The model under review builds one solid part; all positions refer to its coordinate system, in mm. Round coordinates to 2 decimals unless told otherwise and drop trailing zeros. Write each loop counter-clockwise with the first axis right and the second up, starting at its lowest first coordinate (ties: lowest second). Pieces come first, ordered by that corner, then holes.
Item 1: Add section A-A (y = 0). Give the boundary of the cut face in (x, z), plus the area to 3 significant figures.
Item 2: Draft analysis for pull direction Y (two halves, no side actions). For faces 1 (the face through (73.95, 1.651, -5.243)), 2 (the face through (3.45, -6.38, -1.19)), 3 (the face through (73.95, -7.32, 1.63)), state which applies: +Y half, -Y half, draft (parallel to the pull), parting line (faces both ways), or undercut.
Item 3: Add section C-C (x = 24.36). Give the boundary of the cut face in (y, z), plus the area to 3 significant figures.
Item 4: To check wall thickness, follow L1, parallel to X at y = -6.45, z = 0; L2, parallel to X at y = -5.5, z = -1; L3, parallel to Z at x = 121.5, y = -2.5. State the ranges of each line that lie inside material, in increasing order.
Item 5: Add section D-D (x = 112). Give the boundary of the cut face in (y, z), plus the area to 3 significant figures.
Item 6: Add section B-B (z = 0). Give the boundary of the cut face in (x, y), plus the area to 3 significant figures.
```python
from build123d import *

# Parameters (mm, degrees)
SKETCH_1_R          = 7.498521941
SKETCH_1_R_2        = 5.496326061
EXTRUDE_1_DEPTH     = 150
SKETCH_2_R          = 1.5
CUT_EXTRUDE_1_DEPTH = 14


with BuildPart() as part:
    # 草图1 → 凸台-拉伸1 (new body)
    with BuildSketch(Plane(origin=(0, 0, 0), x_dir=(0, 0, -1), z_dir=(1, 0, 0))):
        Circle(SKETCH_1_R)
        Circle(SKETCH_1_R_2, mode=Mode.SUBTRACT)
    extrude(amount=EXTRUDE_1_DEPTH)

    # 草图2 → 切除-拉伸1 (cut, symmetric)
    with BuildSketch(Plane(origin=(0, 0, 0), x_dir=(1, 0, 0), z_dir=(0, 1, 0))):
        with Locations(Location((4.36, 0, 0), (0, 0, 270))):
            Circle(SKETCH_2_R)
        with Locations(Location((24.36, 0, 0), (0, 0, 270))):
            Circle(SKETCH_2_R)
    extrude(amount=CUT_EXTRUDE_1_DEPTH, both=True, mode=Mode.SUBTRACT)


solid = part.part
```
Numbers:
1. outline: (0, -7.5) - (150, -7.5) - (150, -5.5) - (0, -5.5) - close; (0, 5.5) - (150, 5.5) - (150, 7.5) - (0, 7.5) - close
1. area: 601 mm2
2. face 1: undercut
2. face 2: draft
2. face 3: parting line
3. outline: (-7.35, -1.5) arc R7.5 ccw to (7.35, -1.5) - (5.29, -1.5) arc R5.5 cw to (-5.29, -1.5) - close; (-7.35, 1.5) - (-5.29, 1.5) arc R5.5 cw to (5.29, 1.5) - (7.35, 1.5) arc R7.5 ccw to start
3. area: 69.6 mm2
4. L1: x = 0 to 2.86, 5.86 to 22.86, 25.86 to 150
4. L2: x = 0 to 3.24, 5.48 to 23.24, 25.48 to 150
4. L3: z = -7.07 to -4.89, 4.89 to 7.07
5. outline: circle Ø15 at (0, 0); hole circle Ø10.99 at (0, 0)
5. area: 81.7 mm2
6. outline: (0, -7.5) - (2.86, -7.5) - (2.86, -5.5) - (0, -5.5) - close; (0, 5.5) - (2.86, 5.5) - (2.86, 7.5) - (0, 7.5) - close; (5.86, -7.5) - (22.86, -7.5) - (22.86, -5.5) - (5.86, -5.5) - close; (5.86, 5.5) - (22.86, 5.5) - (22.86, 7.5) - (5.86, 7.5) - close; (25.86, -7.5) - (150, -7.5) - (150, -5.5) - (25.86, -5.5) - close; (25.86, 5.5) - (150, 5.5) - (150, 7.5) - (25.86, 7.5) - close
6. area: 577 mm2
